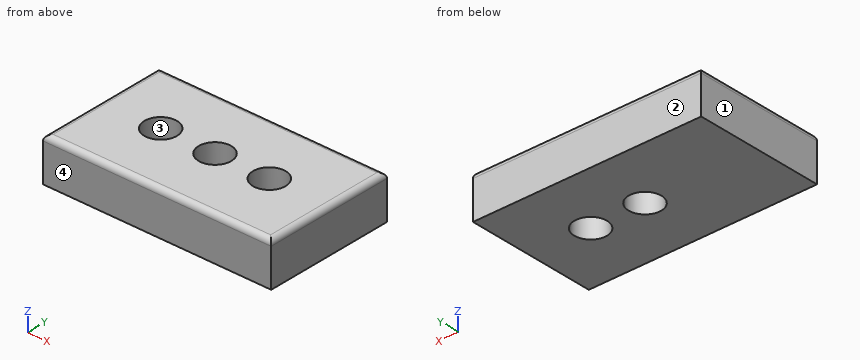
```python
from build123d import *

# Parameters (mm, degrees)
F0_W      = 266.7
F0_H      = 152.4
F1_DEPTH  = 50.8
F2_R      = 19.05
F3_DEPTH  = 38.1
F4_R      = 6.35
F3_FACE_R = 19.05
F5_DEPTH  = 50.8


with BuildPart() as f1:
    # F0 (on Top) → F1 (new body)
    with BuildSketch(Plane.XY):
        Rectangle(F0_W, F0_H)
    extrude(amount=F1_DEPTH)

    # F2 (on face) → F3 (cut)
    with BuildSketch(Plane.XY.offset(50.8)):
        with Locations((-63.5, 0)):
            Circle(F2_R)
        Circle(F2_R)
        with Locations((63.5, 0)):
            Circle(F2_R)
    extrude(amount=-F3_DEPTH, mode=Mode.SUBTRACT)

    # F4
    f4_edges = [f1.edges().sort_by_distance(p)[0] for p in [
        (133.35, 0, 50.8),
        (0, 76.2, 50.8),
        (0, -76.2, 50.8),
        (-133.35, 0, 50.8),
    ]]
    fillet(f4_edges, radius=F4_R)

    # F3_face (on face) → F5 (cut)
    with BuildSketch(Plane.XY.offset(12.7)):
        Circle(F3_FACE_R)
        with Locations((63.5, 0)):
            Circle(F3_FACE_R)
    extrude(amount=-F5_DEPTH, mode=Mode.SUBTRACT)


solid = f1.part
```
Design review of the part built by this model. Coordinates are the model's own, in mm. Face numbers are marked on the shaded views. Round coordinates to 2 decimals unless told otherwise and drop trailing zeros. Write each loop counter-clockwise with the first axis right and the second up, starting at its lowest first coordinate (ties: lowest second). Pieces come first, ordered by that corner, then holes.
Item 1: The part is to be moulded in two halves that separate along Y. For the marked faces 1, 2, 3 and 4, say which applies: +Y half, -Y half, draft (parallel to the pull), parting line (faces both ways), or undercut.
Item 2: We need section A-A on x = 0. Write out the cut boundary in (y, z).
Item 3: Clearance check with a flat-ended pin moving along its axis: pin 1 Ø11.5 at (x, y) = (-60.5, -0.5) entering from +Z. State where the tip first meets the part, or that it passes through.
Item 4: For probe 1 along Y at (x, z) = (63.5, 15.5); probe 2 along Y at (x, z) = (67, 48.5); probe 3 along Z at (x, y) = (-47, -7.5), list the stretches that pass through material, from the lowest coordinate up.
Item 5: We need section C-C on z = 18. Write out the cut boundary in (x, y).
Item 6: We need section B-B on y = 0. Write out the cut boundary in (x, z), and give its area (3 significant figures).
Item 7: We need section D-D on x = -63.5. Write out the cut boundary in (y, z).
Returned:
1. face 1: draft
1. face 2: +Y half
1. face 3: undercut
1. face 4: -Y half
2. outline: (-76.2, 0) - (-19.05, 0) - (-19.05, 50.8) - (-69.85, 50.8) arc R6.35 ccw to (-76.2, 44.45) - close; (19.05, 0) - (76.2, 0) - (76.2, 44.45) arc R6.35 ccw to (69.85, 50.8) - (19.05, 50.8) - close
3. pin 1: stops at z = 12.7
4. probe 1: y = -76.2 to -19.05, 19.05 to 76.2
4. probe 2: y = -74.74 to -18.73, 18.73 to 74.74
4. probe 3: z = 0 to 12.7
5. outline: (-133.35, -76.2) - (133.35, -76.2) - (133.35, 76.2) - (-133.35, 76.2) - close; hole circle Ø38.1 at (-63.5, 0); hole circle Ø38.1 at (0, 0); hole circle Ø38.1 at (63.5, 0)
6. outline: (-133.35, 0) - (-19.05, 0) - (-19.05, 50.8) - (-44.45, 50.8) - (-44.45, 12.7) - (-82.55, 12.7) - (-82.55, 50.8) - (-127, 50.8) arc R6.35 ccw to (-133.35, 44.45) - close; (19.05, 0) - (44.45, 0) - (44.45, 50.8) - (19.05, 50.8) - close; (82.55, 0) - (133.35, 0) - (133.35, 44.45) arc R6.35 ccw to (127, 50.8) - (82.55, 50.8) - close
6. area: 8,210 mm2
7. outline: (-76.2, 0) - (76.2, 0) - (76.2, 44.45) arc R6.35 ccw to (69.85, 50.8) - (19.05, 50.8) - (19.05, 12.7) - (-19.05, 12.7) - (-19.05, 50.8) - (-69.85, 50.8) arc R6.35 ccw to (-76.2, 44.45) - close
